Can you work these out from the model? Positions are in its coordinate system, mm. A direction names the side the tool comes from. Coordinates: 2 decimals unless noted, no trailing zeros. Order: outer loops, then holes, each group sorted by start corner. A loop starts at its lowest first (then second) coordinate and runs counter-clockwise, first axis right, second up. Notation, with made-up numbers: (-29, 47.25) -> (-13, 47.25) arc R27 cw to (-13, 72.25) -> close; hole circle Ø6 at (21.5, 82.25). An arc over 180 degrees is marked (long way). Answer as CSV lines item,"result".
Solid Edge part; units mm, degrees
sketch "Sketch1" plane through (0, 0, 0) normal (0, 0, 1) x (1, 0, 0)
  line L0 (-10, -32.5) -> (10, -32.5)
  line L1 (10, -32.5) -> (10, 32.5)
  line L2 (10, 32.5) -> (-10, 32.5)
  line L3 (-10, 32.5) -> (-10, -32.5)
  circle A0 centre (0, 0) radius 4.6
  dimension "D1" = 10
  dimension "D2" = 10
extrude "Protrusion1" add sketch "Sketch1" along normal blind 4
sketch "Sketch2" plane through (0, 0, 4) normal (0, 0, 1) x (1, 0, 0)
  line L0 (0, 10) -> (10, 10)
  line L1 (10, 10) -> (10, -10)
  line L2 (10, -10) -> (0, -10)
  line L3 (0, -10) -> (0, 10)
  dimension "D1" = 10
extrude "Cutout1" cut sketch "Sketch2" against normal up to next
sketch "Sketch3" plane through (0, 0, 4) normal (0, 0, 1) x (0, 1, 0)
  circle A0 centre (26.5, 0) radius 2.1
  circle A1 centre (-26.5, 0) radius 2.1
extrude "Cutout2" cut sketch "Sketch3" against normal up to next
hole "Hole_1" at (0, 7.3, 2) direction (-1, 0, 0) diameter 1.867 depth 10 thread major 2.3 thread length 8
hole "Hole1" at (0, -7.3, 2) direction (-1, 0, 0) diameter 1.867 depth 10 thread major 2.3 thread length 8
Q1. Imagine slicing it at A-A (x = 3.75). List the corners of the cut face in (y, z) for me, and give its area (3 significant figures).
Solution:
outline,"(-32.5, 0) -> (-10, 0) -> (-10, 4) -> (-32.5, 4) -> close; (10, 0) -> (32.5, 0) -> (32.5, 4) -> (10, 4) -> close"
area,"180 mm2"
Q2. We'd pull the mould along Y, two halves only. Please class faces 3 (the flat face through (0, 32.5, 2)), 4 (the cylindrical face through (-4.6, -0.1, 2)), 5 (the flat face through (-5, 0, 0)), 6 (the flat face through (0, -32.5, 2)): pulls with the +Y half, pulls with the -Y half, needs draft (parallel to the pull), parting line crosses it, or undercut.
Solution:
face 3,"pulls with the +Y half"
face 4,"undercut"
face 5,"needs draft"
face 6,"pulls with the -Y half"
Q3. For P1, Ø1.1, axis at y = -7.3, z = 2, coming from the +X side; P2, Ø1.5, axis at y = -3, z = 0.5, coming from the +X side; P3, Ø1.2, axis at y = 7, z = 3, coming from the +X side, each with a flat end and sliding along its axis, tell me the tip position at first contact or that it passes through.
Solution:
P1,"through"
P2,"x = -2.66"
P3,"x = 0"
Q4. If I drill on line 1 (Y direction, x = -5.5, z = 2); line 2 (Z direction, x = -4, y = -7.3); line 3 (Y direction, x = 8.75, z = 3.35), over which ranges is the centre line in solid material (lowest first)?
Solution:
line 1,"-32.5 to -8.23, -6.37 to 6.37, 8.23 to 32.5"
line 2,"0 to 1.07, 2.93 to 4"
line 3,"-32.5 to -10, 10 to 32.5"
Q5. Imagine slicing it at D-D (y = 0). List the corners of the cut face in (x, z) for me.
Solution:
outline,"(-10, 0) -> (-4.6, 0) -> (-4.6, 4) -> (-10, 4) -> close"
Q6. Which directions (+Z, -Z, +X, -X, +Y, -Y) give clear straight access to the entire face, cutting with the end or side of a thin tool? Please do faces 1 (the flat face through (5, 10, 2)), 2 (the flat face through (-5, 0, 4)).
Solution:
face 1,"+Z, -Z, +X"
face 2,"+Z, +X, -X, +Y, -Y"
Q7. Imagine slicing it at C-C (z = 2.3). List the corners of the cut face in (x, y) for me.
Solution:
outline,"(-10, -32.5) -> (10, -32.5) -> (10, -10) -> (0, -10) -> (0, -8.18) -> (-10, -8.18) -> close; (-10, -6.42) -> (0, -6.42) -> (0, -4.6) arc R4.6 cw to (0, 4.6) -> (0, 6.42) -> (-10, 6.42) -> close; (-10, 8.18) -> (0, 8.18) -> (0, 10) -> (10, 10) -> (10, 32.5) -> (-10, 32.5) -> close; hole circle Ø4.2 at (0, -26.5); hole circle Ø4.2 at (0, 26.5)"
Q8. Imagine slicing it at B-B (y = 26.5). List the corners of the cut face in (x, z) for me.
Solution:
outline,"(-10, 0) -> (-2.1, 0) -> (-2.1, 4) -> (-10, 4) -> close; (2.1, 0) -> (10, 0) -> (10, 4) -> (2.1, 4) -> close"
